Input: part model. Units: mm. Frame: model coordinates. A direction names the side the tool comes from. Round coordinates to 2 decimals unless told otherwise and drop trailing zeros. Loops run counter-clockwise (first coordinate to the right, second up) from the corner with the lowest first, then second, coordinate; pieces in that order, holes last.
1) Ray query, line 1 along X through (y, z) = (-23.5, 19); line 2 along X through (y, z) = (-25, 14); line 3 along Y through (x, z) = (46, 15.5). Return the intervals inside material, ascending.
2) Draft query along Y for faces 3 (the face through (-64, 48, 6.35)), 4 (the face through (76.2, -1, 0)), 5 (the face through (-64, 63.5, 9)), 6 (the face through (-1, 76.2, 0)). Return one class per face: pulls with the +Y half, pulls with the -Y half, needs draft (parallel to the pull), parting line crosses it, or undercut.
3) Access query for faces 1 (the face through (-64, 31.75, 9)), 2 (the face through (46.9, -25.8, -0.4)). Directions: +Z, -Z, +X, -X, +Y, -Y. A direction counts if a zero-diameter tool reaches every point of the face in a straight line with its end or side. Return the directions, or none.
4) Section B-B, the plane y = 60.5. Return loops of the section in (x, z).
5) Section A-A, the plane x = -59. Return loops of the section in (y, z), and give its area (3 significant figures).
from build123d import *

# Parameters (mm, degrees)
F0_W     = 152.4
F0_H     = 50.8
F1_DEPTH = 76.2
F2_R     = 12.7
F4_D     = 6.7564
F5_W     = 31.75
F5_H     = 6.35
F6_DEPTH = 25.4


with BuildPart() as f1:
    # F0 (on Front) → F1 (new body, symmetric)
    with BuildSketch(Plane.XZ):
        Rectangle(F0_W, F0_H)
    extrude(amount=F1_DEPTH, both=True)

    # F2
    f2_edges = [f1.edges().sort_by_distance(p)[0] for p in [
        (0, -76.2, 25.4),
    ]]
    fillet(f2_edges, radius=F2_R)

    # F4 (through all)
    with Locations(Plane.XY.offset(25.4)):
        with Locations((44.2391075194, -23.7217675894)):
            Hole(F4_D / 2)

    # F5 (on face) → F6 (cut)
    with BuildSketch(Plane(origin=(-76.2, 0, 0), x_dir=(0, -1, 0), z_dir=(-1, 0, 0))):
        with Locations((-47.625, 9.525)):
            Rectangle(F5_W, F5_H)
    extrude(amount=-F6_DEPTH, mode=Mode.SUBTRACT)


solid = f1.part
Final values:
1. line 1: x = -76.2 to 40.87, 47.61 to 76.2
1. line 2: x = -76.2 to 41.11, 47.37 to 76.2
1. line 3: y = -75.89 to -26.6, -20.84 to 76.2
2. face 3: undercut
2. face 4: needs draft
2. face 5: undercut
2. face 6: pulls with the +Y half
3. face 1: -X
3. face 2: +Z, -Z
4. outline: (-76.2, -25.4) - (76.2, -25.4) - (76.2, 25.4) - (-76.2, 25.4) - (-76.2, 12.7) - (-50.8, 12.7) - (-50.8, 6.35) - (-76.2, 6.35) - close
5. outline: (-76.2, -25.4) - (76.2, -25.4) - (76.2, 25.4) - (-63.5, 25.4) arc R12.7 ccw to (-76.2, 12.7) - close; hole (31.75, 6.35) - (63.5, 6.35) - (63.5, 12.7) - (31.75, 12.7) - close
5. area: 7,510 mm2
